Model file for the job. Use its own axes, mm. A direction names the side the tool comes from. Coordinates: 2 decimals unless noted, no trailing zeros. Loops run counter-clockwise (first coordinate to the right, second up) from the corner with the lowest first, then second, coordinate; pieces in that order, holes last. Notation, with made-up numbers: (78, 53) -> (91, 53) arc R22 cw to (91, 92) -> close; hole circle Ø11 at (-30, -16.5). An arc over 180 degrees is marked (long way). Use one line per item in the form item = value.
```python
from build123d import *

# Parameters (mm, degrees)
SKETCH_3_R          = 13
EXTRUDE_1_DEPTH     = 5
CUT_EXTRUDE_2_DEPTH = 2.5
SKETCH_6_R          = 2
CUT_EXTRUDE_3_DEPTH = 18
SKETCH_7_R          = 7
CUT_EXTRUDE_4_DEPTH = 8
CUT_EXTRUDE_6_DEPTH = 5
FILLET_1_R          = 1
SKETCH_10_W         = 2
SKETCH_10_H         = 14
CUT_EXTRUDE_7_DEPTH = 0.5


with BuildPart() as part:
    # ｽｹｯﾁ3 → ﾎﾞｽ - 押し出し1 (new body)
    with BuildSketch(Plane.XY):
        Circle(SKETCH_3_R)
    extrude(amount=EXTRUDE_1_DEPTH)

    # ｽｹｯﾁ2 → ｶｯﾄ - 押し出し2 (cut)
    with BuildSketch(Plane.XY):
        with BuildLine():
            Line((3.75, 6.495190528), (2.773808556, 13.582081265))
            ThreePointArc((2.773808556, 13.582081265), (0, 16), (-2.773808556, 13.582081265))
            Line((-2.773808556, 13.582081265), (-3.75, 6.495190528))
            Line((-3.75, 6.495190528), (-10.375523134, 9.193229308))
            ThreePointArc((-10.375523134, 9.193229308), (-13.856406461, 8), (-13.14933169, 4.388851958))
            Line((-13.14933169, 4.388851958), (-7.5, 0))
            Line((-7.5, 0), (-13.14933169, -4.388851958))
            ThreePointArc((-13.14933169, -4.388851958), (-13.856406461, -8), (-10.375523134, -9.193229308))
            Line((-10.375523134, -9.193229308), (-3.75, -6.495190528))
            Line((-3.75, -6.495190528), (-2.773808556, -13.582081265))
            ThreePointArc((-2.773808556, -13.582081265), (0, -16), (2.773808556, -13.582081265))
            Line((2.773808556, -13.582081265), (3.75, -6.495190528))
            Line((3.75, -6.495190528), (10.375523134, -9.193229308))
            ThreePointArc((10.375523134, -9.193229308), (13.856406461, -8), (13.14933169, -4.388851958))
            Line((13.14933169, -4.388851958), (7.5, 0))
            Line((7.5, 0), (13.14933169, 4.388851958))
            ThreePointArc((13.14933169, 4.388851958), (13.856406461, 8), (10.375523134, 9.193229308))
            Line((10.375523134, 9.193229308), (3.75, 6.495190528))
        make_face()
    extrude(amount=CUT_EXTRUDE_2_DEPTH, mode=Mode.SUBTRACT)

    # ｽｹｯﾁ5 → 回転1 (revolve)
    with BuildSketch(Plane(origin=(0, 0, 0), x_dir=(1, 0, 0), z_dir=(0, 1, 0))):
        Polygon((0, -5), (25, -5), (25, -7), (10, -7), (10, -15), (25, -15), (25, -17), (0, -17), align=None)
    revolve(axis=Axis((0, 0, 0), (0, 0, 1)))

    # ｽｹｯﾁ6 → ｶｯﾄ - 押し出し3 (cut, through all)
    with BuildSketch(Plane.XY.offset(17)):
        Circle(SKETCH_6_R)
    extrude(amount=-CUT_EXTRUDE_3_DEPTH, mode=Mode.SUBTRACT)

    # ｽｹｯﾁ7 → ｶｯﾄ - 押し出し4 (cut)
    with BuildSketch(Plane.XY.offset(17)):
        Circle(SKETCH_7_R)
    extrude(amount=-CUT_EXTRUDE_4_DEPTH, mode=Mode.SUBTRACT)

    # ｽｹｯﾁ9 → ｶｯﾄ - 押し出し6 (cut)
    with BuildSketch(Plane(origin=(0, 0, 15), x_dir=(-1, 0, 0), z_dir=(0, 0, -1))):
        Polygon((-3.843473937, -0.691164305), (-11.556925253, -9.883697623), (-7.726703038, -13.097635671), (-0.013251721, -3.905102354), align=None)
    cut_extrude_6 = extrude(amount=CUT_EXTRUDE_6_DEPTH, mode=Mode.SUBTRACT)

    # ﾐﾗｰ1: ｶｯﾄ - 押し出し6 across plane
    add(cut_extrude_6.mirror(Plane(origin=(0, 0, 0), x_dir=(0, 0, 1), z_dir=(1, 0, 0))), mode=Mode.SUBTRACT)

    # ﾌｨﾚｯﾄ1
    fillet_1_edges = [part.edges().sort_by_distance(p)[0] for p in [
        (4.308653161, -9.024162451, 12.5),
        (-4.308653161, -9.024162451, 12.5),
    ]]
    fillet(fillet_1_edges, radius=FILLET_1_R)

    # ｽｹｯﾁ10 → ｶｯﾄ - 押し出し7 (cut)
    with BuildSketch(Plane.XY.offset(17)):
        with Locations((0, 16)):
            Rectangle(SKETCH_10_W, SKETCH_10_H)
    extrude(amount=-CUT_EXTRUDE_7_DEPTH, mode=Mode.SUBTRACT)


solid = part.part
```
Q1. Band-saw the part on A-A, the plane x = 0. Write the cut outline in (y, z), and give its area (3 significant figures).
Result:
outline = (-25, 5) -> (-13, 5) -> (-13, 2.5) -> (-2, 2.5) -> (-2, 9) -> (-7, 9) -> (-7, 17) -> (-25, 17) -> (-25, 15) -> (-10, 15) -> (-10, 7) -> (-25, 7) -> close; (2, 2.5) -> (13, 2.5) -> (13, 5) -> (25, 5) -> (25, 7) -> (10, 7) -> (10, 15) -> (25, 15) -> (25, 17) -> (23, 17) -> (23, 16.5) -> (9, 16.5) -> (9, 17) -> (7, 17) -> (7, 9) -> (2, 9) -> close
area = 280 mm2
Q2. Band-saw the part on B-B, the plane z = 11.5. Write the cut outline in (x, y).
Result:
outline = (-8.14, -5.81) -> (-6.12, -3.4) arc R7 cw (long way) to (6.12, -3.4) -> (8.14, -5.81) arc R10 ccw (long way) to start; (-3.41, -7.96) arc R1 ccw to (-2.94, -9.56) arc R10 ccw to (2.94, -9.56) arc R1 ccw to (3.41, -7.96) -> (2.29, -6.62) arc R7 cw to (-2.29, -6.62) -> close
Q3. Mould opens along Z. For faces 1 (the face through (9.93, 1.89, 1.23)), 2 (the face through (1, 2, 9)), 3 (the face through (7.114, -4.589, 12.535)) say: released by +Z, released by -Z, zero draft, split by the parting line, or undercut.
Result:
face_1 = zero draft
face_2 = released by +Z
face_3 = undercut
Q4. Band-saw the part on C-C, the plane y = 18.5. Write the cut outline in (x, z), and give its area (3 significant figures).
Result:
outline = (-16.82, 5) -> (16.82, 5) -> (16.82, 7) -> (-16.82, 7) -> close; (-16.82, 15) -> (16.82, 15) -> (16.82, 17) -> (1, 17) -> (1, 16.5) -> (-1, 16.5) -> (-1, 17) -> (-16.82, 17) -> close
area = 134 mm2
Q5. Wall check: line 1 along Z through (x, y) = (16, -0.5); line 2 along Y through (x, z) = (0, 14.5); line 3 along Z through (x, y) = (9, -3.5). Give the ranges that are in metal, low to high.
Result:
line_1 = 5 to 7, 15 to 17
line_2 = -10 to -7, 7 to 10
line_3 = 2.5 to 17
Q6. Band-saw the part on D-D, the plane z = 6.25. Write the cut outline in (x, y), and give its area (3 significant figures).
Result:
outline = circle Ø50 at (0, 0); hole circle Ø4 at (0, 0)
area = 1,950 mm2
Q7. Pin check, flat tips, straight feed: pin 1 Ø2 at (y, z) = (13.5, 6) entering from +X; pin 2 Ø25 at (x, y) = (4, 10) entering from -Z; pin 3 Ø5 at (x, y) = (3, -19.5) entering from -Z; pin 4 Ø0.6 at (x, z) = (0, 17) entering from +Y. Stop position of each tip, or through.
Result:
pin_1 = 21.65
pin_2 = 0
pin_3 = 5
pin_4 = 25
Q8. Which spindle directions (+Z, -Z, +X, -X, +Y, -Y) get a long thin tool onto all of the face, cutting with end or side? Do faces 4 (the face through (-6.68, -7.69, 1.23)), 5 (the face through (-11, -11, 5)), 6 (the face through (0, 16, 16.5)). Say none if no direction does.
Result:
face_4 = -Z, -X
face_5 = -Z
face_6 = +Z
